Geometry: final body of the model. Coordinates: model frame, mm. Coordinates: 2 decimals unless noted, no trailing zeros. Write each loop counter-clockwise with the first axis right and the second up, starting at its lowest first coordinate (ties: lowest second). Pieces come first, ordered by that corner, then holes. Notation, with made-up numbers: M -39.5,9.5 L 15.5,9.5 A21 ccw 15.5,23.5 Z; hole C 48,-27 d3. An arc over 180 degrees is marked long. Write item = value, one per line. Start each with the question number.
Item 1: Section C-C on y = 0.75. Give the number of separate pieces and of enclosed holes in the cut face, plus the area to 3 significant figures.
Item 2: Ray query, L1, parallel to X at y = 2.1, z = 20.5; L2, parallel to Z at x = -27.5, y = 0.9; L3, parallel to X at y = 0.3, z = 25.5. Return the intervals inside material, ascending. Write a range as [from, to].
Item 3: Section A-A on x = -18.5. Output: boundary loops of the cut face in (y, z).
Item 4: Section B-B on z = -3.5. Output: boundary loops of the cut face in (x, y), plus the area to 3 significant figures.
from build123d import *

# Parameters (mm, degrees)
SKETCH1_W           = 372
SKETCH1_H           = 104.22
BOSS_EXTRUDE1_DEPTH = 4.7625
SKETCH2_R           = 2
CUT_EXTRUDE1_DEPTH  = 10
SKETCH3_R           = 2
CUT_EXTRUDE2_DEPTH  = 10
CUT_EXTRUDE3_DEPTH  = 26
SKETCH5_W           = 62.455838456
SKETCH5_H           = 25.297024562
CUT_EXTRUDE4_DEPTH  = 10
FILLET2_SIZE        = 5


with BuildPart() as part:
    # Sketch1 → Boss-Extrude1 (new body)
    with BuildSketch(Plane(origin=(0, 0, 0), x_dir=(1, 0, 0), z_dir=(0, 1, 0))):
        with Locations((72.169818201, 7.186191072)):
            Rectangle(SKETCH1_W, SKETCH1_H)
    extrude(amount=BOSS_EXTRUDE1_DEPTH)

    # Sketch2 → Cut-Extrude1 (cut)
    with BuildSketch(Plane(origin=(0, 4.7625, 0), x_dir=(1, 0, 0), z_dir=(0, 1, 0))):
        with BuildLine():
            ThreePointArc((-107.830181799, 39.296191072), (-108.415968237, 40.710404634), (-109.830181799, 41.296191072))
            Line((-109.830181799, 41.296191072), (-109.830181799, 39.296191072))
            Line((-109.830181799, 39.296191072), (-111.830181799, 39.296191072))
            ThreePointArc((-111.830181799, 39.296191072), (-109.830181799, 37.296191072), (-107.830181799, 39.296191072))
        make_face()
        with BuildLine():
            Line((-109.830181799, 39.296191072), (-109.830181799, 41.296191072))
            ThreePointArc((-109.830181799, 41.296191072), (-111.244395361, 40.710404634), (-111.830181799, 39.296191072))
            Line((-111.830181799, 39.296191072), (-109.830181799, 39.296191072))
        make_face()
        with BuildLine():
            ThreePointArc((256.169818201, 39.296191072), (255.584031763, 40.710404634), (254.169818201, 41.296191072))
            Line((254.169818201, 41.296191072), (254.169818201, 39.296191072))
            Line((254.169818201, 39.296191072), (256.169818201, 39.296191072))
        make_face()
        with BuildLine():
            Line((254.169818201, 39.296191072), (254.169818201, 41.296191072))
            ThreePointArc((254.169818201, 41.296191072), (252.755604639, 37.88197751), (256.169818201, 39.296191072))
            Line((256.169818201, 39.296191072), (254.169818201, 39.296191072))
        make_face()
        with Locations(Location((-109.830181799, -24.923808928, 0), (0, 0, 270))):
            Circle(SKETCH2_R)
        with Locations(Location((254.169818201, -24.923808928, 0), (0, 0, 270))):
            Circle(SKETCH2_R)
    extrude(amount=-CUT_EXTRUDE1_DEPTH, mode=Mode.SUBTRACT)

    # Sketch3 → Cut-Extrude2 (cut)
    with BuildSketch(Plane(origin=(0, 4.7625, 0), x_dir=(1, 0, 0), z_dir=(0, 1, 0))):
        with Locations(Location((72.169818201, 39.296191072, 0), (0, 0, 270))):
            Circle(SKETCH3_R)
        with Locations(Location((72.169818201, -24.923808928, 0), (0, 0, 270))):
            Circle(SKETCH3_R)
    extrude(amount=-CUT_EXTRUDE2_DEPTH, mode=Mode.SUBTRACT)

    # Sketch4 → Cut-Extrude3 (cut)
    with BuildSketch(Plane(origin=(0, 4.7625, 0), x_dir=(1, 0, 0), z_dir=(0, 1, 0))):
        with BuildLine():
            ThreePointArc((92.169818201, 7.186191072), (86.311953825, 21.328326696), (72.169818201, 27.186191072))
            Line((72.169818201, 27.186191072), (72.169818201, -12.813808928))
            ThreePointArc((72.169818201, -12.813808928), (86.311953825, -6.955944552), (92.169818201, 7.186191072))
        make_face()
        with BuildLine():
            Line((72.169818201, -12.813808928), (72.169818201, 27.186191072))
            ThreePointArc((72.169818201, 27.186191072), (52.169818201, 7.186191072), (72.169818201, -12.813808928))
        make_face()
    extrude(amount=-CUT_EXTRUDE3_DEPTH, mode=Mode.SUBTRACT)

    # Sketch5 → Cut-Extrude4 (cut)
    with BuildSketch(Plane(origin=(0, 4.7625, 0), x_dir=(1, 0, 0), z_dir=(0, 1, 0))):
        with Locations((-0.819204667, -22.766901993)):
            Rectangle(SKETCH5_W, SKETCH5_H)
        with Locations((145.158841069, -22.766901993)):
            Rectangle(SKETCH5_W, SKETCH5_H)
    extrude(amount=-CUT_EXTRUDE4_DEPTH, mode=Mode.SUBTRACT)

    # Fillet2
    # a fillet whose section is not a circle: 5 mm, written as the material it adds along each edge
    with BuildSketch(Plane(origin=(176.386760297, 4.7625, 35.415414274), x_dir=(0, 0, -1), z_dir=(0, -1, 0)), Plane(origin=(113.930921841, 4.7625, 10.118389712), x_dir=(0, 0, 1), z_dir=(0, -1, 0)), Plane(origin=(113.930921841, 4.7625, 35.415414274), x_dir=(1, 0, 0), z_dir=(0, -1, 0)), Plane(origin=(30.408714561, 4.7625, 35.415414274), x_dir=(0, 0, -1), z_dir=(0, -1, 0)), Plane(origin=(30.408714561, 4.7625, 10.118389712), x_dir=(-1, 0, 0), z_dir=(0, -1, 0)), Plane(origin=(-32.047123895, 4.7625, 35.415414274), x_dir=(1, 0, 0), z_dir=(0, -1, 0))) as fillet2_piece_1:
        with BuildLine():
            add(Edge.make_bspline([(FILLET2_SIZE, 0), (FILLET2_SIZE * 0.831801948466, 0), (FILLET2_SIZE * 0.663603896932, 0), (FILLET2_SIZE * 0.292893218813, -FILLET2_SIZE * 0.0716919198361), (FILLET2_SIZE * 0.0716919198361, -FILLET2_SIZE * 0.292893218813), (0, -FILLET2_SIZE * 0.663603896932), (0, -FILLET2_SIZE * 0.831801948466), (0, -FILLET2_SIZE)], knots=[0, 0, 0, 0, 0, 0, 0.5, 0.5, 1, 1, 1, 1, 1, 1], degree=5))
            Line((0, -FILLET2_SIZE), (-FILLET2_SIZE * 0.02, -FILLET2_SIZE))
            Line((-FILLET2_SIZE * 0.02, -FILLET2_SIZE), (-FILLET2_SIZE * 0.02, FILLET2_SIZE * 0.02))
            Line((-FILLET2_SIZE * 0.02, FILLET2_SIZE * 0.02), (FILLET2_SIZE, FILLET2_SIZE * 0.02))
            Line((FILLET2_SIZE, FILLET2_SIZE * 0.02), (FILLET2_SIZE, 0))
        make_face()
    extrude(amount=4.7625)
    with BuildSketch(Plane(origin=(176.386760297, 4.7625, 10.118389712), x_dir=(0, 0, 1), z_dir=(0, -1, 0)), Plane(origin=(-32.047123895, 4.7625, 10.118389712), x_dir=(1, 0, 0), z_dir=(0, -1, 0))) as fillet2_piece_2:
        with BuildLine():
            add(Edge.make_bspline([(FILLET2_SIZE, 0), (FILLET2_SIZE * 0.831801948466, 0), (FILLET2_SIZE * 0.663603896932, 0), (FILLET2_SIZE * 0.292893218813, FILLET2_SIZE * 0.0716919198361), (FILLET2_SIZE * 0.0716919198361, FILLET2_SIZE * 0.292893218813), (0, FILLET2_SIZE * 0.663603896932), (0, FILLET2_SIZE * 0.831801948466), (0, FILLET2_SIZE)], knots=[0, 0, 0, 0, 0, 0, 0.5, 0.5, 1, 1, 1, 1, 1, 1], degree=5))
            Line((0, FILLET2_SIZE), (-FILLET2_SIZE * 0.02, FILLET2_SIZE))
            Line((-FILLET2_SIZE * 0.02, FILLET2_SIZE), (-FILLET2_SIZE * 0.02, -FILLET2_SIZE * 0.02))
            Line((-FILLET2_SIZE * 0.02, -FILLET2_SIZE * 0.02), (FILLET2_SIZE, -FILLET2_SIZE * 0.02))
            Line((FILLET2_SIZE, -FILLET2_SIZE * 0.02), (FILLET2_SIZE, 0))
        make_face()
    extrude(amount=4.7625)


solid = part.part
Responses:
q1.separate_pieces = 1
q1.enclosed_holes = 9
q1.area = 34,300 mm²
q2.L1 = [-113.83, -32.05], [30.41, 113.93], [176.39, 258.17]
q2.L2 = [-59.3, 10.12], [35.41, 44.92]
q2.L3 = [-113.83, -111.75], [-107.91, -32.05], [30.41, 70.25], [74.09, 113.93], [176.39, 252.25], [256.09, 258.17]
q3.outline = M 0,-59.3 L 4.76,-59.3 L 4.76,10.12 L 0,10.12 Z; M 0,35.42 L 4.76,35.42 L 4.76,44.92 L 0,44.92 Z
q4.outline = M -113.83,0 L 52.51,0 L 52.51,4.76 L -113.83,4.76 Z; M 91.83,0 L 258.17,0 L 258.17,4.76 L 91.83,4.76 Z
q4.area = 1,580 mm²
